```python
from build123d import *

# Parameters (mm, degrees)
F1_DEPTH = 6
F2_W     = 5.5
F2_H     = 10
F3_DEPTH = 25
F4_R     = 1.5
F5_DEPTH = 6


with BuildPart() as f1:
    # F0 (on Top) → F1 (new body)
    with BuildSketch(Plane.XY):
        with BuildLine():
            Line((-30.5, -42.5), (30.5, -42.5))
            ThreePointArc((30.5, -42.5), (31.914214, -41.914214), (32.5, -40.5))
            Line((32.5, -40.5), (32.5, 40.5))
            ThreePointArc((32.5, 40.5), (31.914214, 41.914214), (30.5, 42.5))
            Line((30.5, 42.5), (-30.5, 42.5))
            ThreePointArc((-30.5, 42.5), (-31.914214, 41.914214), (-32.5, 40.5))
            Line((-32.5, 40.5), (-32.5, -40.5))
            ThreePointArc((-32.5, -40.5), (-31.914214, -41.914214), (-30.5, -42.5))
        make_face()
    extrude(amount=F1_DEPTH)

    # F2 (on face) → F3 (cut)
    with BuildSketch(Plane.XY.offset(6)):
        with Locations((-25, 25)):
            Rectangle(F2_W, F2_H)
        with Locations((25, 25)):
            Rectangle(F2_W, F2_H)
        with Locations((25, -25)):
            Rectangle(F2_W, F2_H)
        with Locations((-25, -25)):
            Rectangle(F2_W, F2_H)
    extrude(amount=-F3_DEPTH, mode=Mode.SUBTRACT)

    # F4 (on face) → F5 (cut)
    with BuildSketch(Plane.XY.offset(6)):
        with Locations((-12.5, 38)):
            Circle(F4_R)
        with Locations((12.5, 38)):
            Circle(F4_R)
        with Locations((12.5, -38)):
            Circle(F4_R)
        with Locations((-12.5, -38)):
            Circle(F4_R)
    extrude(amount=-F5_DEPTH, mode=Mode.SUBTRACT)


solid = f1.part
```
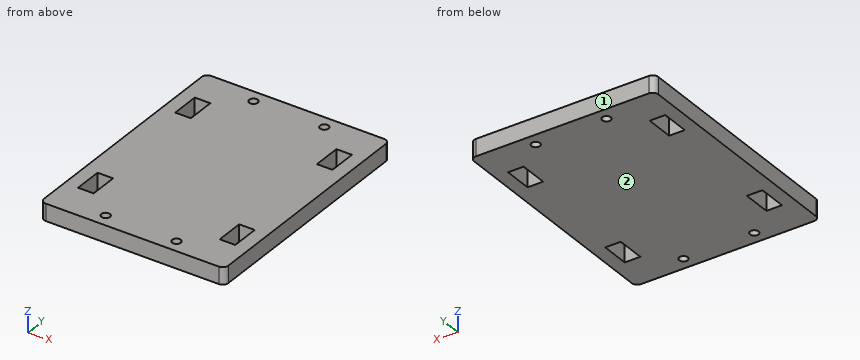
Source: CAD feature listing. Evaluate the final solid. Frame: model axes, mm. Face numbers are marked on the shaded views. Coordinates: 2 decimals unless noted, no trailing zeros. Write each loop counter-clockwise with the first axis right and the second up, starting at its lowest first coordinate (ties: lowest second). Pieces come first, ordered by that corner, then holes. Notation, with made-up numbers: (18, 47.25) -> (32, 47.25) arc R16 cw to (32, 56.25) -> close; hole circle Ø5 at (19.5, 13.5). An arc over 180 degrees is marked (long way). Return JSON: item names as keys, results as strings. Group by question number.
1) Contact query for flat-ended pins moving along their axis: P1, Ø1.8, axis at x = -12.5, y = 38, coming from the -Z side; P2, Ø4, axis at x = -12.5, y = -38, coming from the +Z side. Output: stop coordinate, or through.
2) Mould query, pull axis Y, two halves, no side actions, for the marked faces 1 and 2. Classes: +Y half, -Y half, draft (parallel to the pull), parting line (faces both ways), or undercut.
3) Section query B-B, the plane y = 38. Return loops of the section in (x, z).
4) Section query C-C, the plane z = 1.25. State how many separate pieces and enclosed holes the cut face has, plus the area to 3 significant figures.
5) Section query A-A, the plane x = 12.5. Return loops of the section in (y, z).
6) Ray query, line 1 along Y through (x, z) = (24.5, 2.1); line 2 along Y through (x, z) = (-12.5, 4.15); line 3 along X through (y, z) = (22, 3.35). Return the intervals inside material, ascending.
From the geometry:
{
 "1": {"P1": "through", "P2": "z = 6"},
 "2": {"face 1": "+Y half", "face 2": "draft"},
 "3": {"outline": "(-32.5, 0) -> (-14, 0) -> (-14, 6) -> (-32.5, 6) -> close; (-11, 0) -> (11, 0) -> (11, 6) -> (-11, 6) -> close; (14, 0) -> (32.5, 0) -> (32.5, 6) -> (14, 6) -> close"},
 "4": {"separate pieces": "1", "enclosed holes": "8", "area": "5,270 mm²"},
 "5": {"outline": "(-42.5, 0) -> (-39.5, 0) -> (-39.5, 6) -> (-42.5, 6) -> close; (-36.5, 0) -> (36.5, 0) -> (36.5, 6) -> (-36.5, 6) -> close; (39.5, 0) -> (42.5, 0) -> (42.5, 6) -> (39.5, 6) -> close"},
 "6": {"line 1": "-42.5 to -30, -20 to 20, 30 to 42.5", "line 2": "-42.5 to -39.5, -36.5 to 36.5, 39.5 to 42.5", "line 3": "-32.5 to -27.75, -22.25 to 22.25, 27.75 to 32.5"}
}
